Here's how the part is built. I have some questions about the finished solid (model axes, mm). Face numbers are marked on the shaded views. A direction names the side the tool comes from. Give positions to 0.01 mm unless a question says otherwise; leave off trailing zeros. Loops run counter-clockwise (first coordinate to the right, second up) from the corner with the lowest first, then second, coordinate; pieces in that order, holes last.
Q1. Suppose I cut it at C-C (y = 7.5). List the corners of the cut face in (x, z) for me, and give its area (3 significant figures).
Q2. I need wall thicknesses on probe 1 along Z at (x, y) = (0, 7.75); probe 2 along X at (y, z) = (10, -85.5); probe 3 along Y at (x, z) = (14, 15.5). Which ranges of each line are inside material? Lowest first, please.
Q3. Suppose I cut it at B-B (z = -80.5). List the corners of the cut face in (x, y) for me, and give its area (3 significant figures).
Q4. Suppose I cut it at D-D (y = 28). List the corners of the cut face in (x, z) for me.
Q5. I'm going to push flat-ended pins straight in: P1, Ø15, axis at x = -1, z = -21.5, coming from the -Y side; P2, Ø1.5, axis at x = 0.5, z = 150.5, coming from the -Y side; P3, Ø8, axis at x = 3.5, z = -22.5, coming from the +Y side. Where does each tip first touch, or does it pass through?
Q6. Suppose I cut it at A-A (x = 0). List the corners of the cut face in (y, z) for me.
Q7. For the marked faces 1, 2 and 3, which set-ups out of +Z, -Z, +X, -X, +Y, -Y let a thin tool reach every point of the face, with its end or its side?
```python
from build123d import *

# Parameters (mm, degrees)
F0_W     = 40
F0_H     = 300
F1_DEPTH = 25
F2_R     = 15
F3_DEPTH = 10
F4_R     = 5
F5_R     = 4.99999
F6_R     = 22.5487204306
F7_DEPTH = 25


# Not quite as in the source:
# - a fillet or chamfer is up to 0.001 mm smaller than in the source, because OpenCascade refuses the exact size


with BuildPart() as f1:
    # F0 (on Front) → F1 (new body)
    with BuildSketch(Plane.XZ):
        with Locations((0, 32.5)):
            Rectangle(F0_W, F0_H)
    extrude(amount=-F1_DEPTH)

    # F2 (on Front) → F3 (cut)
    with BuildSketch(Plane.XZ):
        with Locations((0, 147.7966460525)):
            Circle(F2_R)
    extrude(amount=-F3_DEPTH, mode=Mode.SUBTRACT)

    # F4
    f4_edges = [f1.edges().sort_by_distance(p)[0] for p in [
        (20, 25, 32.5),
        (-20, 25, 32.5),
        (0, 25, 182.5),
    ]]
    fillet(f4_edges, radius=F4_R)

    # F5 (radius 5 in the source; OpenCascade refuses exactly that, so slightly less here)
    f5_edges = [f1.edges().sort_by_distance(p)[0] for p in [
        (20, 0, 32.5),
        (-20, 0, 32.5),
        (0, 0, 182.5),
    ]]
    fillet(f5_edges, radius=F5_R)

    # F6 (on face) → F7 (join)
    with BuildSketch(Plane(origin=(0, 0, -117.5), x_dir=(1, 0, 0), z_dir=(0, 0, -1))):
        with Locations((0, -13.4554868564)):
            Circle(F6_R)
    extrude(amount=-F7_DEPTH)


solid = f1.part
```
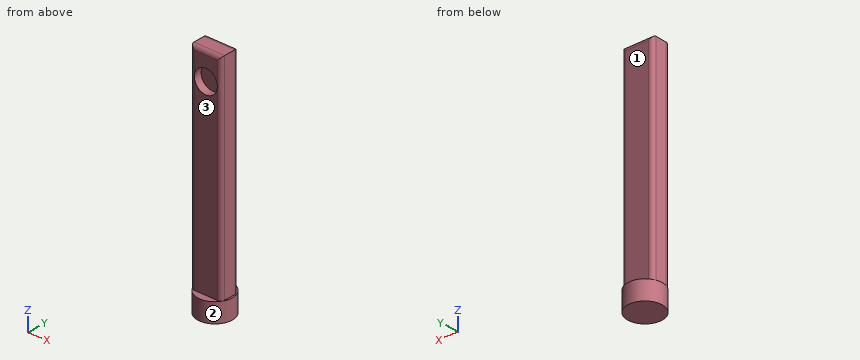
Solutions:
1. outline: (-21.75, -117.5) - (21.75, -117.5) - (21.75, -92.5) - (20, -92.5) - (20, 182.5) - (-20, 182.5) - (-20, -92.5) - (-21.75, -92.5) - close; hole circle Ø30 at (0, 147.8)
1. area: 11,400 mm2
2. probe 1: z = -117.5 to 132.8, 162.8 to 182.5
2. probe 2: x = -20 to 20
2. probe 3: y = 0 to 25
3. outline: (-20, 5) arc R5 ccw to (-15, 0) - (15, 0) arc R5 ccw to (20, 5) - (20, 20) arc R5 ccw to (15, 25) - (-15, 25) arc R5 ccw to (-20, 20) - close
3. area: 979 mm2
4. outline: (-17.23, -117.5) - (17.23, -117.5) - (17.23, -92.5) - (-17.23, -92.5) - close
5. P1: stops at y = 0
5. P2: stops at y = 10
5. P3: stops at y = 25
6. outline: (-9.09, -117.5) - (36, -117.5) - (36, -92.5) - (25, -92.5) - (25, 177.5) arc R5 ccw to (20, 182.5) - (5, 182.5) arc R5 ccw to (0, 177.5) - (0, 162.8) - (10, 162.8) - (10, 132.8) - (0, 132.8) - (0, -92.5) - (-9.09, -92.5) - close
7. face 1: +Z, +X, -X, +Y
7. face 2: +Z, -Z
7. face 3: +Z, +X, -X, -Y
